Autodesk Inventor part; units mm, degrees
ref_plane "YZ Plane" through (0, 0, 0) normal (1, 0, 0) x (0, 1, 0)
ref_plane "XZ Plane" through (0, 0, 0) normal (0, 1, 0) x (-1, 0, 0)
ref_plane "XY Plane" through (0, 0, 0) normal (0, 0, 1) x (1, 0, 0)
sketch "Sketch1" plane through (0, 0, 0) normal (0, 1, 0) x (-1, 0, 0)
  line L0 (2, 0) -> (65, 0)
  line L1 (67, -2) -> (67, -90)
  line L2 (65, -92) -> (2, -92)
  line L3 (0, -90) -> (0, -2)
  arc A0 (67, -2) -> (65, 0) centre (65, -2) ccw
  arc A1 (65, -92) -> (67, -90) centre (65, -90) ccw
  arc A2 (0, -90) -> (2, -92) centre (2, -90) ccw
  arc A3 (2, 0) -> (0, -2) centre (2, -2) ccw
  line L4 (8, -8) -> (59, -8)
  line L5 (59, -84) -> (8, -84)
  line L6 (59, -8) -> (59, -32.2523)
  line L7 (59, -59.7477) -> (59, -84)
  line L8 (8, -84) -> (8, -59.7477)
  line L9 (8, -32.2523) -> (8, -8)
  arc A4 (59, -59.7477) -> (59, -32.2523) centre (33.5, -46) ccw
  arc A5 (8, -32.2523) -> (8, -59.7477) centre (33.5, -46) ccw
  circle A6 centre (62.4698, -4) radius 2
  circle A7 centre (62.4698, -87) radius 2
  circle A8 centre (4.5302, -4) radius 2
  circle A9 centre (4.5302, -87) radius 2
  point P0 (0, 0)
  point P1 (67, -92)
  point P2 (67, 0)
  point P3 (0, -92)
  dimension "d40" = 67
  dimension "d41" = 92
  dimension "d42" = 2
  dimension "d43" = 51
  dimension "d44" = 76
extrude "Extrusion9" add sketch "Sketch1" along normal blind 1
Check sheet for the modelled part. Datum: model origin and axes. Units: mm. A direction names the side the tool comes from. Coordinates: 2 decimals unless noted, no trailing zeros. Order: outer loops, then holes, each group sorted by start corner. A loop starts at its lowest first (then second) coordinate and runs counter-clockwise, first axis right, second up. Notation, with made-up numbers: M 43,-28 L 62,-28 A8 cw 62,-19 Z; hole C -37.5,84 d6. An arc over 180 degrees is marked long. One line per question, with ' | ' between items. Start each with the question number.
Item 1: Gauge pin test, flat end, axial feed: P1, Ø3, axis at x = -4.53, z = -4, coming from the +Y side. Record the tip position at first contact, or that the pin passes through.
Item 2: Sectioned sample at C-C on z = -15.5. Record the cut outline in (x, y), and give its area (3 significant figures).
Item 3: Sectioned sample at D-D on y = 0.4. Record the cut outline in (x, z), and give its area (3 significant figures).
Item 4: Sectioned sample at B-B on z = -4. Record the cut outline in (x, y).
Item 5: Access from +Z, -Z, +X, -X, +Y, -Y to the whole of each face (thin tool, end or side, straight path). Record for faces 4 (the cylindrical face through (-62.47, 0.49, -45.8)), 5 (the cylindrical face through (-66.43, 0.49, -91.4)).
Item 6: Material ranges on line 1 (X direction, y = 0.6, z = -73); line 2 (Z direction, x = -32, y = 0.8); line 3 (Z direction, x = -64, y = 0.4), recorded low to high.
Item 7: Mould release check, pull along X, two halves, no side actions. Record for faces 1 (the cylindrical face through (-60.47, 0.49, -4.09)), 2 (the flat face through (-61, 1, -36)), 3 (the cylindrical face through (-0.57, 0.49, -0.6)): pulls with the +X half, pulls with the -X half, needs draft (parallel to the pull), parting line crosses it, or undercut.
Item 8: Sectioned sample at A-A on x = -31. Record the cut outline in (y, z).
Answer below:
1) P1: passes through
2) outline: M -67,0 L -59,0 L -59,1 L -67,1 Z; M -8,0 L 0,0 L 0,1 L -8,1 Z | area: 16.0 mm^2
3) outline: M -67,-90 A2 ccw -65,-92 L -2,-92 A2 ccw 0,-90 L 0,-2 A2 ccw -2,0 L -65,0 A2 ccw -67,-2 Z; hole C -62.47,-87 d4; hole C -62.47,-4 d4; hole M -59,-84 L -8,-84 L -8,-59.75 A28.97 ccw -8,-32.25 L -8,-8 L -59,-8 L -59,-32.25 A28.97 ccw -59,-59.75 Z; hole C -4.53,-87 d4; hole C -4.53,-4 d4 | area: 2,110 mm^2
4) outline: M -67,0 L -64.47,0 L -64.47,1 L -67,1 Z; M -60.47,0 L -6.53,0 L -6.53,1 L -60.47,1 Z; M -2.53,0 L 0,0 L 0,1 L -2.53,1 Z
5) face 4: +Y, -Y | face 5: -Z, -X, +Y, -Y
6) line 1: x = -67 to -59, -8 to 0 | line 2: z = -92 to -84, -8 to 0 | line 3: z = -92 to -88.29, -85.71 to -5.29, -2.71 to 0
7) face 1: undercut | face 2: needs draft | face 3: pulls with the +X half
8) outline: M 0,-92 L 1,-92 L 1,-84 L 0,-84 Z; M 0,-8 L 1,-8 L 1,0 L 0,0 Z
